Here's how the part is built. I have some questions about the finished solid (model axes, mm). Round coordinates to 2 decimals unless told otherwise and drop trailing zeros. Answer in a Markdown table with one row per item. Add a question column.
from build123d import *

# Parameters (mm, degrees)
F0_R     = 76.2
F1_DEPTH = 6.35
F2_R     = 73.025
F3_DEPTH = 3.175
F5_R     = 12.7


# Not quite as in the source:
# - a fillet or chamfer that OpenCascade refuses, or shapes differently, is made with other operations: its cross-section is extruded or revolved along the edge and cut away or added


with BuildPart() as f1:
    # F0 (on Top) → F1 (new body)
    with BuildSketch(Plane.XY):
        Circle(F0_R)
    extrude(amount=F1_DEPTH)

    # F2 (on face) → F3 (cut)
    with BuildSketch(Plane.XY.offset(6.35)):
        Circle(F2_R)
    extrude(amount=-F3_DEPTH, mode=Mode.SUBTRACT)

    # F4: fillet of radius 1.5875 on 2 edges, made by hand

    # F4_s1 → F4_t2 (revolve, cut)
    with BuildSketch(Plane.XZ):
        with BuildLine():
            ThreePointArc((74.6125, 6.35), (73.4899679849, 5.8850320151), (73.025, 4.7625))
            Line((73.025, 4.7625), (73.025, 6.35))
            Line((73.025, 6.35), (74.6125, 6.35))
        make_face()
    revolve(axis=Axis((0, 0, 6.35), (0, 0, 1)), mode=Mode.SUBTRACT)

    # F4_s3 → F4_t4 (revolve, cut)
    with BuildSketch(Plane.XZ):
        with BuildLine():
            ThreePointArc((76.2, 4.7625), (75.7350320151, 5.8850320151), (74.6125, 6.35))
            Line((74.6125, 6.35), (76.2, 6.35))
            Line((76.2, 6.35), (76.2, 4.7625))
        make_face()
    revolve(axis=Axis((0, 0, 6.35), (0, 0, 1)), mode=Mode.SUBTRACT)

    # F5
    f5_edges = [f1.edges().sort_by_distance(p)[0] for p in [
        (-73.025, 0, 3.175),
    ]]
    fillet(f5_edges, radius=F5_R)

    # F6: fillet of radius 25.4 on 1 edges, made by hand

    # F6_s1 → F6_t2 (revolve, cut)
    with BuildSketch(Plane.XZ):
        with BuildLine():
            ThreePointArc((76.2, 4.7625), (69.1699156866, 1.2199203889), (61.3927857532, 0))
            Line((61.3927857532, 0), (61.3927857532, -0.508))
            Line((61.3927857532, -0.508), (76.2, -0.508))
            Line((76.2, -0.508), (76.708, 0))
            ThreePointArc((76.708, 0), (76.708, 2.38125), (76.4961442849, 4.34975))
            Line((76.4961442849, 4.34975), (76.2, 4.7625))
        make_face()
    revolve(axis=Axis((0, 0, 0), (0, 0, 1)), mode=Mode.SUBTRACT)


solid = f1.part
Item 1: If we mould it in two halves opening along X, with no side actions, what happens to faces 1 (the flat face through (-1, 1, 0)), 2 (the flat face through (-1, 1, 3.175))? For each: pulls with the +X half, pulls with the -X half, needs draft (parallel to the pull), parting line crosses it, or undercut.
Item 2: I need wall thicknesses on line 1 along Z through (x, y) = (9.5, -49) (3 decimals); line 2 along X through (y, z) = (30, 5.5); line 3 along X through (y, z) = (-5, 5.5). Which ranges of each line are inside material? Lowest first, please. Write a range as from..to.
Item 3: For P1, Ø3, axis at y = 21.5, z = 3, coming from the +X side; P2, Ø1.5, axis at x = 58, z = 5.5, coming from the +Y side; P3, Ø1.5, axis at x = 45.5, y = -46, coming from the +Z side (3 decimals), each with a flat end and sliding along its axis, tell me the tip position at first contact or that it passes through.
Results list:
| question | item | result |
|---|---|---|
| 1 | face 1 | needs draft |
| 1 | face 2 | undercut |
| 2 | line 1 | 0..3.175 |
| 2 | line 2 | -69.85..-66.5, 66.5..69.85 |
| 2 | line 3 | -75.85..-72.79, 72.79..75.85 |
| 3 | P1 | x = 72.76 |
| 3 | P2 | y = 50.12 |
| 3 | P3 | z = 3.175 |
